The listing builds one solid part. Answer for the finished solid, in the listing's coordinates (mm). Face numbers are marked on the shaded views. A direction names the side the tool comes from. Round coordinates to 2 decimals unless told otherwise and drop trailing zeros. Write each loop counter-clockwise with the first axis right and the second up, starting at its lowest first coordinate (ties: lowest second). Pieces come first, ordered by that corner, then holes. Notation, with made-up numbers: M 61,-18.5 L 98,-18.5 A28 cw 98,15.5 Z; hole C -21.75,36.5 d7. An arc over 180 degrees is marked long. One line per item, written item: value. Start each with the question number.
(1) Consider probe 1 along X at (y, z) = (5, -10.5); probe 2 along Y at (x, z) = (-84, -35) (3 decimals); probe 3 along X at (y, z) = (27, 9). Determine where each line is inside the solid, lowest interval first.
(2) Given P1, Ø10.5, axis at x = -62.5, z = -42.5, coming from the +Y side; P2, Ø3, axis at y = 36, z = -3.5, coming from the +X side; P3, Ø1.5, axis at x = 50, y = 5.5, coming from the +Z side, each flat-ended and moving along its own axis, determine where each tip first touches the part or whether it passes through.
(3) Section B-B (x = -62.3) is taken. Determine the outline of the cut face in (y, z) (3 decimals).
(4) For a pull along Z with two mould halves and no side action, classify the marked faces 6, 7 and 8 as released by +Z, released by -Z, zero draft, split by the parting line, or undercut.
(5) For the marked faces 1, 2, 3, 4 and 5, determine the directions among +Z, -Z, +X, -X, +Y, -Y from which every point of the face is accessible in a straight line to the end or side of a thin tool.
(6) Section A-A (y = 32) is taken. Determine the outline of the cut face in (x, z) (3 decimals), plus the area to 3 significant figures.
```python
from build123d import *

# Parameters (mm, degrees)
BOSS_EXTRUDE1_DEPTH = 4
FILLET1_R           = 4
SKETCH4_W           = 4
SKETCH4_H           = 4
SKETCH4_H_2         = 100
BOSS_EXTRUDE2_DEPTH = 50
BOSS_EXTRUDE3_DEPTH = 25
BOSS_EXTRUDE4_DEPTH = 12
SKETCH5_3_W         = 8
SKETCH5_3_H         = 8
CUT_EXTRUDE1_DEPTH  = 12
SKETCH6_W           = 79
SKETCH6_H           = 50
CUT_EXTRUDE2_DEPTH  = 1
SKETCH6_3_W         = 81
SKETCH6_3_H         = 56
SKETCH6_3_W_2       = 79
SKETCH6_3_H_2       = 50
BOSS_EXTRUDE5_DEPTH = 3
SKETCH7_R           = 4.175
BOSS_EXTRUDE6_DEPTH = 50
CUT_EXTRUDE3_START  = 50
SKETCH7_2_R         = 2.175
CUT_EXTRUDE3_DEPTH  = 5
SKETCH9_R           = 4.675
SKETCH9_R_2         = 2.175
BOSS_EXTRUDE7_DEPTH = 5
SKETCH10_R          = 4.675
SKETCH10_R_2        = 2.175
BOSS_EXTRUDE8_DEPTH = 5


with BuildPart() as part:
    # Sketch1 → Boss-Extrude1 (new body)
    with BuildSketch(Plane(origin=(0, 0, 0), x_dir=(1, 0, 0), z_dir=(0, 1, 0))):
        with BuildLine():
            Line((-88.5, -54), (88.5, -54))
            ThreePointArc((88.5, -54), (91.328427125, -52.828427125), (92.5, -50))
            Line((92.5, -50), (92.5, 50))
            ThreePointArc((92.5, 50), (91.328427125, 52.828427125), (88.5, 54))
            Line((88.5, 54), (-88.5, 54))
            ThreePointArc((-88.5, 54), (-91.328427125, 52.828427125), (-92.5, 50))
            Line((-92.5, 50), (-92.5, -50))
            ThreePointArc((-92.5, -50), (-91.328427125, -52.828427125), (-88.5, -54))
        make_face()
    extrude(amount=BOSS_EXTRUDE1_DEPTH)

    # Fillet1
    fillet1_edges = [part.edges().sort_by_distance(p)[0] for p in [
        (0, 0, 54),
        (91.328427125, 0, 52.828427125),
        (92.5, 0, 0),
        (91.328427125, 0, -52.828427125),
        (0, 0, -54),
        (-91.328427125, 0, -52.828427125),
        (-92.5, 0, 0),
        (-91.328427125, 0, 52.828427125),
    ]]
    fillet(fillet1_edges, radius=FILLET1_R - 0.0001)  # a hair under: the kernel refuses the full size

    # Sketch4 → Boss-Extrude2 (add)
    with BuildSketch(Plane(origin=(0, 4, 0), x_dir=(1, 0, 0), z_dir=(0, 1, 0))):
        with BuildLine():
            ThreePointArc((-92.5, -50), (-91.328427125, -52.828427125), (-88.5, -54))
            Line((-88.5, -54), (-8.5, -54))
            Line((-8.5, -54), (-8.5, -50))
            Line((-8.5, -50), (-88.5, -50))
            Line((-88.5, -50), (-88.5, 50))
            Line((-88.5, 50), (-8.5, 50))
            Line((-8.5, 50), (-8.5, 54))
            Line((-8.5, 54), (-88.5, 54))
            ThreePointArc((-88.5, 54), (-91.328427125, 52.828427125), (-92.5, 50))
            Line((-92.5, 50), (-92.5, -50))
        make_face()
        with Locations((-6.5, 52)):
            Rectangle(SKETCH4_W, SKETCH4_H)
        with Locations((-6.5, 0)):
            Rectangle(SKETCH4_W, SKETCH4_H_2)
        with Locations((-6.5, -52)):
            Rectangle(SKETCH4_W, SKETCH4_H)
    extrude(amount=BOSS_EXTRUDE2_DEPTH)

    # Sketch4<3> → Boss-Extrude3 (add)
    with BuildSketch(Plane(origin=(0, 4, 0), x_dir=(1, 0, 0), z_dir=(0, 1, 0))):
        Polygon((-0.5, 50), (-0.5, -50), (3.5, -50), (3.5, -46), (3.5, 46), (3.5, 50), align=None)
        Polygon((3.5, -46), (3.5, -50), (88.5, -50), (88.5, 50), (3.5, 50), (3.5, 46), (84.5, 46), (84.5, -46), align=None)
    extrude(amount=BOSS_EXTRUDE3_DEPTH)

    # Sketch5 → Boss-Extrude4 (add)
    with BuildSketch(Plane.ZY.offset(8.5)):
        Polygon((-46, 4), (-42, 4), (-42, 12), (-34, 12), (-34, 4), (-30, 4), (-30, 16), (-46, 16), align=None)
    extrude(amount=-BOSS_EXTRUDE4_DEPTH)

    # Sketch5<3> → Cut-Extrude1 (cut)
    with BuildSketch(Plane.ZY.offset(8.5)):
        with Locations((-38, 8)):
            Rectangle(SKETCH5_3_W, SKETCH5_3_H)
    extrude(amount=-CUT_EXTRUDE1_DEPTH, mode=Mode.SUBTRACT)

    # Sketch6 → Cut-Extrude2 (cut)
    with BuildSketch(Plane(origin=(0, 4, 0), x_dir=(1, 0, 0), z_dir=(0, 1, 0))):
        with Locations((44, 0)):
            Rectangle(SKETCH6_W, SKETCH6_H)
    extrude(amount=-CUT_EXTRUDE2_DEPTH, mode=Mode.SUBTRACT)

    # Sketch6<3> → Boss-Extrude5 (add)
    with BuildSketch(Plane(origin=(0, 4, 0), x_dir=(1, 0, 0), z_dir=(0, 1, 0))):
        with Locations((44, 0)):
            Rectangle(SKETCH6_3_W, SKETCH6_3_H)
        with Locations((44, 0)):
            Rectangle(SKETCH6_3_W_2, SKETCH6_3_H_2, mode=Mode.SUBTRACT)
    extrude(amount=BOSS_EXTRUDE5_DEPTH)

    # Sketch7 → Boss-Extrude6 (add)
    with BuildSketch(Plane(origin=(0, 4, 0), x_dir=(1, 0, 0), z_dir=(0, 1, 0))):
        with Locations((-86.962042751, 48.462042751)):
            Circle(SKETCH7_R)
        with Locations((-10.037957249, 48.462042751)):
            Circle(SKETCH7_R)
        with Locations((-10.037957249, -48.462042751)):
            Circle(SKETCH7_R)
        with Locations((-86.962042751, -48.462042751)):
            Circle(SKETCH7_R)
    extrude(amount=BOSS_EXTRUDE6_DEPTH)

    # Sketch7<2> → Cut-Extrude3 (cut)
    with BuildSketch(Plane(origin=(0, 4, 0), x_dir=(1, 0, 0), z_dir=(0, 1, 0)).offset(CUT_EXTRUDE3_START)):
        with Locations(Location((-86.962042751, 48.462042751, 0), (0, 0, 270))):
            Circle(SKETCH7_2_R)
        with Locations(Location((-10.037957249, 48.462042751, 0), (0, 0, 270))):
            Circle(SKETCH7_2_R)
        with Locations(Location((-10.037957249, -48.462042751, 0), (0, 0, 270))):
            Circle(SKETCH7_2_R)
        with Locations(Location((-86.962042751, -48.462042751, 0), (0, 0, 270))):
            Circle(SKETCH7_2_R)
    extrude(amount=-CUT_EXTRUDE3_DEPTH, mode=Mode.SUBTRACT)

    # Sketch9 → Boss-Extrude7 (add)
    # profile 1 of 4: a face of its own
    with BuildSketch(Plane(origin=(0, 4, 0), x_dir=(1, 0, 0), z_dir=(0, 1, 0))):
        with Locations(Location((-62.3, 43.75, 0), (0, 0, 90))):
            Circle(SKETCH9_R)
        with Locations(Location((-62.3, 43.75, 0), (0, 0, 270))):
            Circle(SKETCH9_R_2, mode=Mode.SUBTRACT)
    # profile 2 of 4: a face of its own
    with BuildSketch(Plane(origin=(0, 4, 0), x_dir=(1, 0, 0), z_dir=(0, 1, 0))):
        with Locations(Location((-20.3, 43.75, 0), (0, 0, 90))):
            Circle(SKETCH9_R)
        with Locations(Location((-20.3, 43.75, 0), (0, 0, 270))):
            Circle(SKETCH9_R_2, mode=Mode.SUBTRACT)
    # profile 3 of 4: a face of its own
    with BuildSketch(Plane(origin=(0, 4, 0), x_dir=(1, 0, 0), z_dir=(0, 1, 0))):
        with Locations(Location((-62.3, -16.25, 0), (0, 0, 90))):
            Circle(SKETCH9_R)
        with Locations(Location((-62.3, -16.25, 0), (0, 0, 270))):
            Circle(SKETCH9_R_2, mode=Mode.SUBTRACT)
    # profile 4 of 4: a face of its own
    with BuildSketch(Plane(origin=(0, 4, 0), x_dir=(1, 0, 0), z_dir=(0, 1, 0))):
        with Locations(Location((-20.3, -16.25, 0), (0, 0, 90))):
            Circle(SKETCH9_R)
        with Locations(Location((-20.3, -16.25, 0), (0, 0, 270))):
            Circle(SKETCH9_R_2, mode=Mode.SUBTRACT)
    extrude(amount=BOSS_EXTRUDE7_DEPTH)

    # Sketch10 → Boss-Extrude8 (add)
    # profile 1 of 4: a face of its own
    with BuildSketch(Plane(origin=(-88.5, 0, 0), x_dir=(0, 0, -1), z_dir=(1, 0, 0))):
        with Locations((-14, 47)):
            Circle(SKETCH10_R)
        with Locations((-14, 47)):
            Circle(SKETCH10_R_2, mode=Mode.SUBTRACT)
    # profile 2 of 4: a face of its own
    with BuildSketch(Plane(origin=(-88.5, 0, 0), x_dir=(0, 0, -1), z_dir=(1, 0, 0))):
        with Locations((35, 47)):
            Circle(SKETCH10_R)
        with Locations((35, 47)):
            Circle(SKETCH10_R_2, mode=Mode.SUBTRACT)
    # profile 3 of 4: a face of its own
    with BuildSketch(Plane(origin=(-88.5, 0, 0), x_dir=(0, 0, -1), z_dir=(1, 0, 0))):
        with Locations((35, 11)):
            Circle(SKETCH10_R)
        with Locations((35, 11)):
            Circle(SKETCH10_R_2, mode=Mode.SUBTRACT)
    # profile 4 of 4: a face of its own
    with BuildSketch(Plane(origin=(-88.5, 0, 0), x_dir=(0, 0, -1), z_dir=(1, 0, 0))):
        with Locations((-14, 11)):
            Circle(SKETCH10_R)
        with Locations((-14, 11)):
            Circle(SKETCH10_R_2, mode=Mode.SUBTRACT)
    extrude(amount=BOSS_EXTRUDE8_DEPTH)


solid = part.part
```
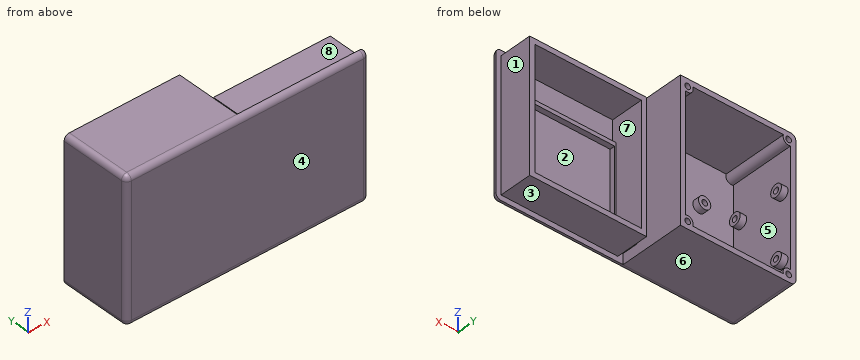
Recorded:
1. probe 1: x = -92.5 to -88.5, -8.5 to -4.5, -0.5 to 4.5, 83.5 to 88.5
1. probe 2: y = 0 to 4, 6.325 to 8.825, 13.175 to 15.675, 42.325 to 44.825, 49.175 to 51.675
1. probe 3: x = -92.5 to -88.5, -8.5 to -4.5, -0.5 to 3.5, 84.5 to 88.5
2. P1: stops at y = 9
2. P2: stops at x = -4.5
2. P3: stops at z = 50
3. outline: M 0,-50 A4 ccw 4,-54 L 54,-54 L 54,-50 L 4,-50 L 4,-48.425 L 9,-48.425 L 9,-45.925 L 4,-45.925 L 4,-41.575 L 9,-41.575 L 9,-39.075 L 4,-39.075 L 4,11.575 L 9,11.575 L 9,14.075 L 4,14.075 L 4,18.425 L 9,18.425 L 9,20.925 L 4,20.925 L 4,50 L 54,50 L 54,54 L 4,54 A4 ccw 0,50 Z
4. face 6: released by -Z
4. face 7: undercut
4. face 8: released by +Z
5. face 1: +Z, -Z, +X, +Y
5. face 2: +Y
5. face 3: -Z, +X, +Y
5. face 4: +Z, -Z, +X, -X, -Y
5. face 5: none
6. outline: M -92.5,-50 A4 ccw -88.5,-54 L -4.5,-54 L -4.5,54 L -88.5,54 A4 ccw -92.5,50 Z; hole M -88.5,-44.581 A4.175 cw -83.081,-50 L -13.919,-50 A4.175 cw -8.5,-44.581 L -8.5,44.581 A4.175 cw -13.919,50 L -83.081,50 A4.175 cw -88.5,44.581 Z
6. area: 1,610 mm2
